Here's how the part is built. I have some questions about the finished solid (model axes, mm). Face numbers are marked on the shaded views. A direction names the side the tool comes from. Round coordinates to 2 decimals unless told otherwise and drop trailing zeros. Write each loop counter-clockwise with the first axis right and the second up, starting at its lowest first coordinate (ties: lowest second). Pieces come first, ordered by that corner, then holes. Notation, with made-up numbers: M 39.25,39 L 71.25,39 A17 ccw 71.25,47 Z; hole C 86.5,27 d11. An arc over 180 degrees is marked long. Use one line per item in the form item = value. Start each with the question number.
Q1. I want a section at C-C on y = 2.75. List the corners of the cut face in (x, z) for me.
Q2. We'd pull the mould along Z, two halves only. Please class the marked faces 4, 5 and 6: +Z half, -Z half, draft (parallel to the pull), parting line (faces both ways), or undercut.
Q3. I want a section at B-B on y = 7.25. List the corners of the cut face in (x, z) for me.
Q4. I need wall thicknesses on line 1 along Z through (x, y) = (0, 5.05); line 2 along X through (y, z) = (6.75, -0.5); line 3 along Z through (x, y) = (1.25, 4.5). Which ranges of each line are inside material? Lowest first, please. Write a range as from..to.
Q5. For the marked faces 1, 2 and 3, which set-ups out of +Z, -Z, +X, -X, +Y, -Y let a thin tool reach every point of the face, with its end or its side?
Q6. I'm going to push flat-ended pins straight in: pin 1 Ø4 at (x, y) = (-1.5, 6) entering from +Z; pin 2 Ø3 at (x, y) = (3, 4.5) entering from +Z; pin 3 Ø3.5 at (x, z) = (0.5, 0.5) entering from +Y. Where does each tip first touch, or does it pass through?
Autodesk Inventor part; units mm, degrees
ref_plane "YZ Plane" through (0, 0, 0) normal (1, 0, 0) x (0, 1, 0)
ref_plane "XZ Plane" through (0, 0, 0) normal (0, 1, 0) x (-1, 0, 0)
ref_plane "XY Plane" through (0, 0, 0) normal (0, 0, 1) x (1, 0, 0)
sketch "Sketch1" plane through (0, 0, 0) normal (0, 0, 1) x (1, 0, 0)
  line L0 (0, 0) -> (-1.6, 0) construction
  line L1 (0, 0) -> (0, 8)
  line L2 (-1.6, 0) -> (-4.6, 0)
  line L3 (-1.6, 0) -> (-1.6, 3.5)
  line L4 (-1.6, 3.5) -> (-3.1, 3.5)
  line L5 (-3.1, 3.5) -> (-3.1, 8)
  line L6 (-3.1, 8) -> (-4.6, 8)
  line L7 (-4.6, 8) -> (-4.6, 4)
  line L8 (-4.6, 4) -> (-3.6, 4)
  line L9 (-3.6, 4) -> (-3.6, 2.5)
  line L10 (-3.6, 2.5) -> (-4.6, 2.5)
  line L11 (-4.6, 2.5) -> (-4.6, 0)
  dimension "d0" = 1.6
  dimension "d1" = 8
  dimension "d2" = 3
  dimension "d3" = 3.5
  dimension "d4" = 1.5
  dimension "d5" = 4
  dimension "d6" = 1
  dimension "d7" = 1.5
revolve "Revolution1" add sketch "Sketch1" angle 360 about axis through (0, 0, 0) along (0, 1, 0)
chamfer "Chamfer1" distance 1 angle 45 2 edges at (4.6, 2.5, 0) (4.6, 4, 0)
chamfer "Chamfer2" distance 0.25 angle 45 4 edges at (4.6, 8, 0) (3.1, 8, 0) (4.6, 0, 0) (1.6, 0, 0)
properties part number "Z25_Side_Lock_Button" material "Aluminum 6061"
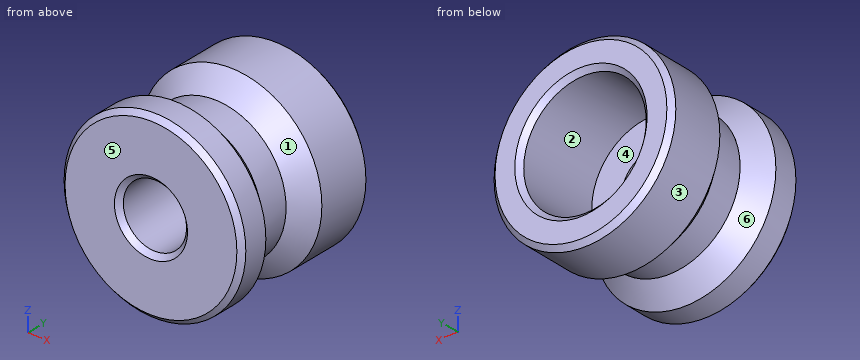
Reported:
q1.outline = C 0,0 d7.2; hole C 0,0 d3.2
q2.face_4 = undercut
q2.face_5 = draft
q2.face_6 = parting line
q3.outline = C 0,0 d9.2; hole C 0,0 d6.2
q4.line_1 = -4.6..-3.1, 3.1..4.6
q4.line_2 = -4.57..-3.06, 3.06..4.57
q4.line_3 = -3.91..-2.84, 2.84..3.91
q5.face_1 = none
q5.face_2 = +Y
q5.face_3 = +Y, -Y
q6.pin_1 = 4.6
q6.pin_2 = 4.32
q6.pin_3 = 3.5
